Input: part model. Units: mm. Frame: model coordinates. Face numbers are marked on the shaded views. Round coordinates to 2 decimals unless told otherwise and drop trailing zeros. Write each loop counter-clockwise with the first axis right and the second up, starting at its lowest first coordinate (ties: lowest second). Pieces come first, ordered by that corner, then holes. Notation, with made-up numbers: M 39,45.5 L 96,45.5 A18 cw 96,70.5 Z; hole C 29,29 d4. An arc over 180 degrees is marked long. Write each question's results on one line, items separated by ' | '. Start each with the question number.
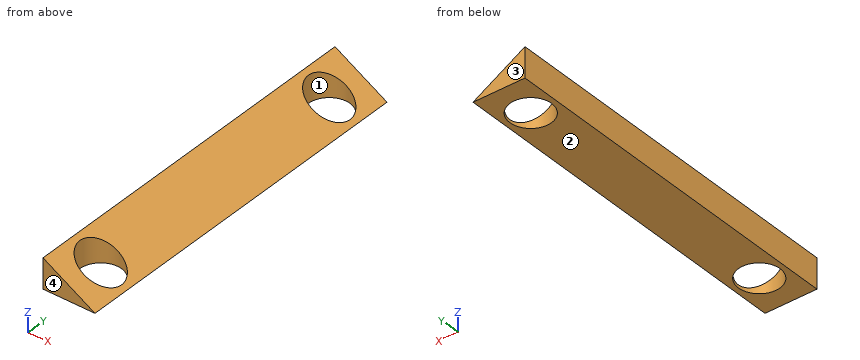
```python
from build123d import *

# Parameters (mm, degrees)
F1_DEPTH = 28
F3_D     = 3
F3_DEPTH = 14.4
F2_R     = 1.6
F4_DEPTH = 25


with BuildPart() as f1:
    # F0 (on Front) → F1 (new body)
    with BuildSketch(Plane.XZ):
        Polygon((0, 2.309401), (0, 0), (4, 0), align=None)
    extrude(amount=F1_DEPTH)

    # F3
    with Locations(Plane(origin=(0, 0, 0), x_dir=(1, 0, 0), z_dir=(0, 0, -1))):
        with Locations((2, 24.956)):
            Hole(F3_D / 2, depth=F3_DEPTH)

    # F2 (on face) → F4 (cut)
    with BuildSketch(Plane(origin=(0, 0, 0), x_dir=(1, 0, 0), z_dir=(0, 0, -1))):
        with Locations((2, 24.956)):
            Circle(F2_R)
        with Locations((2, 3.044)):
            Circle(F2_R)
    extrude(amount=-F4_DEPTH, mode=Mode.SUBTRACT)


solid = f1.part
```
1. Cut plane B-B on x = 2. Output: boundary loops of the cut face in (y, z), and give its area (3 significant figures).
2. Line query: L1, parallel to Y at x = 2, z = 0.75; L2, parallel to Y at x = 1.5, z = 0.45; L3, parallel to Z at x = 3.3, y = -14. Output: solid intervals per line, ascending. Write a range as from..to.
3. Draft query along Y for the marked faces 1, 2, 3 and 4. Return one class per face: +Y half, -Y half, draft (parallel to the pull), parting line (faces both ways), or undercut.
4. Cut plane C-C on z = 1.55. Output: boundary loops of the cut face in (x, y).
5. Cut plane A-A on y = -25.75. Output: boundary loops of the cut face in (x, z), and give its area (3 significant figures).
6. Cut plane D-D on x = 3.05. Output: boundary loops of the cut face in (y, z), and give its area (3 significant figures).
Answers follow:
1) outline: M -28,0 L -26.56,0 L -26.56,1.15 L -28,1.15 Z; M -23.36,0 L -4.64,0 L -4.64,1.15 L -23.36,1.15 Z; M -1.44,0 L 0,0 L 0,1.15 L -1.44,1.15 Z | area: 24.9 mm2
2) L1: y = -28..-26.56, -23.36..-4.64, -1.44..0 | L2: y = -28..-26.48, -23.44..-4.56, -1.52..0 | L3: z = 0..0.4
3) face 1: undercut | face 2: draft | face 3: +Y half | face 4: -Y half
4) outline: M 0,-28 L 1.32,-28 L 1.32,-26.4 A1.6 cw 1.32,-23.51 L 1.32,-4.49 A1.6 cw 1.32,-1.6 L 1.32,0 L 0,0 Z
5) outline: M 0,0 L 0.61,0 L 0.61,1.96 L 0,2.31 Z; M 3.39,0 L 4,0 L 3.39,0.35 Z | area: 1.41 mm2
6) outline: M -28,0 L -26.16,0 L -26.16,0.55 L -28,0.55 Z; M -23.75,0 L -4.25,0 L -4.25,0.55 L -23.75,0.55 Z; M -1.84,0 L 0,0 L 0,0.55 L -1.84,0.55 Z | area: 12.7 mm2
